Read the model definition and answer for the solid it produces. Units are mm, in the model's axes. Coordinates: 2 decimals unless noted, no trailing zeros. Write each loop counter-clockwise with the first axis right and the second up, starting at its lowest first coordinate (ties: lowest second). Pieces come first, ordered by that corner, then holes. Notation, with made-up numbers: (-15.75, 46.5) -> (28.25, 46.5) arc R10 ccw to (28.25, 63.5) -> close; hole circle Ø4 at (-19, 57). An arc over 180 degrees is marked (long way). Write item = value, one per line. Start each with the question number.
1) Section A-A (x = 49) is taken. Determine the outline of the cut face in (y, z), plus the area to 3 significant figures.
2) Flat-ended cylindrical pins translate along their axes: pin 1 Ø1.5 at (y, z) = (4, 3) entering from -X; pin 2 Ø0.7 at (x, z) = (29.5, -5) entering from -Y; pin 3 Ø6 at (x, y) = (66.5, 30) entering from +Z. Find the tip coordinate at first contact, or state that the pin passes through.
3) Find the intervals of material crossed by line 1 along Y through (x, z) = (41, 0); line 2 along Z through (x, y) = (92, 40); line 3 along X through (y, z) = (83, 2.5), in increasing order. Write a range as from..to.
4) Section B-B (y = -2.5) is taken. Determine the outline of the cut face in (x, z), plus the area to 3 significant figures.
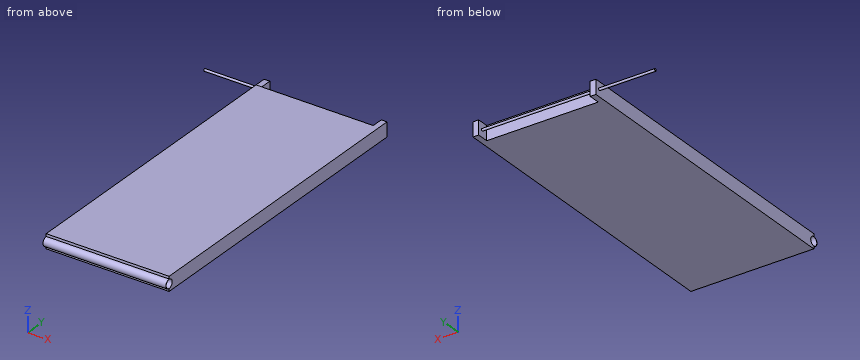
from build123d import *

# Parameters (mm, degrees)
ESQUISSE1_W             = 12.5
ESQUISSE1_H             = 262.5
BOSS_EXTRU_1_DEPTH      = 107.5
ESQUISSE5_R             = 4
BOSS_EXTRU_2_DEPTH      = 107.5
ESQUISSE6_R             = 3.8
ENL_V_MAT_EXTRU_1_DEPTH = 108.5
ESQUISSE8_W             = 5
ESQUISSE8_H             = 12.552801664
BOSS_EXTRU_3_DEPTH      = 10
ESQUISSE9_W             = 5
ESQUISSE9_H             = 12.5
BOSS_EXTRU_4_DEPTH      = 10
BOSS_EXTRU_5_DEPTH      = 101
BOSS_EXTRU_5_DEPTH_BACK = 54
ESQUISSE12_R            = 1


with BuildPart() as part:
    # Esquisse1 → Boss.-Extru.1 (new body)
    with BuildSketch(Plane(origin=(0, 0, 0), x_dir=(0, 0, -1), z_dir=(1, 0, 0))):
        Rectangle(ESQUISSE1_W, ESQUISSE1_H)
    extrude(amount=BOSS_EXTRU_1_DEPTH)

    # Esquisse5 → Boss.-Extru.2 (add)
    with BuildSketch(Plane(origin=(107.5, 0, 0), x_dir=(0, 0, -1), z_dir=(1, 0, 0))):
        with Locations((0, -131.25)):
            Circle(ESQUISSE5_R)
    extrude(amount=-BOSS_EXTRU_2_DEPTH)

    # Esquisse6 → Enlèv. mat.-Extru.1 (cut)
    with BuildSketch(Plane(origin=(107.5, 0, 0), x_dir=(0, 0, -1), z_dir=(1, 0, 0))):
        with Locations((0, -131.179209748)):
            Circle(ESQUISSE6_R)
    extrude(amount=-ENL_V_MAT_EXTRU_1_DEPTH, mode=Mode.SUBTRACT)

    # Esquisse8 → Boss.-Extru.3 (add)
    with BuildSketch(Plane(origin=(0, 131.25, 0), x_dir=(1, 0, 0), z_dir=(0, 1, 0))):
        with Locations((2.5, -0.026400832)):
            Rectangle(ESQUISSE8_W, ESQUISSE8_H)
    extrude(amount=BOSS_EXTRU_3_DEPTH)

    # Esquisse9 → Boss.-Extru.4 (add)
    with BuildSketch(Plane(origin=(0, 131.25, 0), x_dir=(1, 0, 0), z_dir=(0, 1, 0))):
        with Locations((105, 0)):
            Rectangle(ESQUISSE9_W, ESQUISSE9_H)
    extrude(amount=BOSS_EXTRU_4_DEPTH)

    # Esquisse12 → Boss.-Extru.5 (add, two sides: drawn at the far end of the back side and taken through both)
    with BuildSketch(Plane(origin=(5, 0, 0), x_dir=(0, 0, -1), z_dir=(1, 0, 0)).offset(-BOSS_EXTRU_5_DEPTH_BACK)):
        with Locations((0.03, 136.944722229)):
            Circle(ESQUISSE12_R)
    extrude(amount=BOSS_EXTRU_5_DEPTH + BOSS_EXTRU_5_DEPTH_BACK)


solid = part.part
Answer key:
q1.outline = (-131.25, -6.25) -> (131.25, -6.25) -> (131.25, 6.25) -> (-131.25, 6.25) -> (-131.25, 4) arc R4 ccw to (-131.25, -4) -> close; circle Ø2 at (136.94, -0.03); hole circle Ø7.6 at (-131.18, 0)
q1.area = 3,260 mm^2
q2.pin_1 = 0
q2.pin_2 = -131.25
q2.pin_3 = 6.25
q3.line_1 = -135.25..-134.98, -127.38..131.25, 135.95..137.94
q3.line_2 = -6.25..6.25
q3.line_3 = 0..107.5
q4.outline = (0, -6.25) -> (107.5, -6.25) -> (107.5, 6.25) -> (0, 6.25) -> close
q4.area = 1,340 mm^2
